Verification items for the finished model (mm, model axes). A direction names the side the tool comes from. Coordinates: 2 decimals unless noted, no trailing zeros. Write each loop counter-clockwise with the first axis right and the second up, starting at its lowest first coordinate (ties: lowest second). Pieces come first, ordered by that corner, then holes. Notation, with made-up numbers: M 5.25,-33 L 43.25,-33 A31 cw 43.25,-7 Z; hole C -26,-12.5 d4. An arc over 180 degrees is marked long. Answer in a Markdown table with one row per item.
from build123d import *

# Parameters (mm, degrees)
PAD_DEPTH       = 40
POCKET_DEPTH    = 35
POCKET001_DEPTH = 5
FILLET_R        = 0.5
FILLET001_R     = 0.5
CHAMFER_SIZE    = 1


with BuildPart() as part:
    # Sketch → Pad (new body)
    with BuildSketch(Plane.XY):
        with BuildLine():
            Line((-25, 20), (25, 20))
            ThreePointArc((30, 15), (28.535534, 18.535534), (25, 20))
            Line((30, 15), (30, -15))
            ThreePointArc((25, -20), (28.535534, -18.535534), (30, -15))
            Line((25, -20), (-25, -20))
            ThreePointArc((-30, -15), (-28.535534, -18.535534), (-25, -20))
            Line((-30, -15), (-30, 15))
            ThreePointArc((-25, 20), (-28.535534, 18.535534), (-30, 15))
        make_face()
    extrude(amount=PAD_DEPTH)

    # Sketch001 (on Face10 of Pad) → Pocket (cut)
    with BuildSketch(Plane.XY.offset(40)):
        with BuildLine():
            Line((-22.5, 17.5), (22.5, 17.5))
            ThreePointArc((27.5, 12.5), (26.035534, 16.035534), (22.5, 17.5))
            Line((27.5, 12.5), (27.5, -12.5))
            ThreePointArc((22.5, -17.5), (26.035534, -16.035534), (27.5, -12.5))
            Line((22.5, -17.5), (-22.5, -17.5))
            ThreePointArc((-27.5, -12.5), (-26.035534, -16.035534), (-22.5, -17.5))
            Line((-27.5, -12.5), (-27.5, 12.5))
            ThreePointArc((-22.5, 17.5), (-26.035534, 16.035534), (-27.5, 12.5))
        make_face()
    extrude(amount=-POCKET_DEPTH, mode=Mode.SUBTRACT)

    # Sketch002 (on Face6 of Pocket) → Pocket001 (cut)
    with BuildSketch(Plane.XZ.offset(20)):
        with BuildLine():
            Line((-13.5, 40), (13.5, 40))
            Line((13.5, 40), (13.5, 28.982013))
            ThreePointArc((11, 26.482013), (12.767767, 27.214246), (13.5, 28.982013))
            Line((11, 26.482013), (-11, 26.482013))
            ThreePointArc((-13.5, 28.982013), (-12.767767, 27.214246), (-11, 26.482013))
            Line((-13.5, 28.982013), (-13.5, 40))
        make_face()
    extrude(amount=-POCKET001_DEPTH, mode=Mode.SUBTRACT)

    # Fillet
    fillet_edges = [part.edges().sort_by_distance(p)[0] for p in [
        (13.5, -17.5, 34.491006),
        (12.767767, -17.5, 27.214246),
        (0, -17.5, 26.482013),
        (-12.767767, -17.5, 27.214246),
        (-13.5, -17.5, 34.491006),
        (-18, -17.5, 40),
        (-26.035534, -16.035534, 40),
        (-27.5, 0, 40),
        (-26.035534, 16.035534, 40),
        (0, 17.5, 40),
        (26.035534, 16.035534, 40),
        (27.5, 0, 40),
        (26.035534, -16.035534, 40),
        (18, -17.5, 40),
    ]]
    fillet(fillet_edges, radius=FILLET_R)

    # Fillet001
    fillet001_edges = [part.edges().sort_by_distance(p)[0] for p in [
        (-19.25, -20, 40),
        (-13.5, -20, 34.491006),
        (-12.767767, -20, 27.214246),
        (0, -20, 26.482013),
        (12.767767, -20, 27.214246),
        (13.5, -20, 34.491006),
        (19.25, -20, 40),
        (28.535534, -18.535534, 40),
        (30, 0, 40),
        (28.535534, 18.535534, 40),
        (0, 20, 40),
        (-28.535534, 18.535534, 40),
        (-30, 0, 40),
        (-28.535534, -18.535534, 40),
    ]]
    fillet(fillet001_edges, radius=FILLET001_R)

    # Chamfer
    chamfer_edges = [part.edges().sort_by_distance(p)[0] for p in [
        (0, -20, 0),
        (28.535534, -18.535534, 0),
        (30, 0, 0),
        (28.535534, 18.535534, 0),
        (0, 20, 0),
        (-28.535534, 18.535534, 0),
        (-30, 0, 0),
        (-28.535534, -18.535534, 0),
    ]]
    chamfer(chamfer_edges, length=CHAMFER_SIZE)


solid = part.part
1) Release check for a two-part mould opening along Y. For faces 4 (the face through (0, 0, 0)), 5 (the face through (-26.07, -16, 22.49)), 6 (the face through (-29, -18, 20)) record: +Y half, -Y half, draft (parallel to the pull), parting line (faces both ways), or undercut.
Response values:
| item | result |
|---|---|
| face 4 | draft |
| face 5 | undercut |
| face 6 | -Y half |
2) Sectioned sample at A-A (z = 20). Record the cut outline in (x, y), then the cut area to 3 significant figures.
Response values:
| item | result |
|---|---|
| outline | M -30,-15 A5 ccw -25,-20 L 25,-20 A5 ccw 30,-15 L 30,15 A5 ccw 25,20 L -25,20 A5 ccw -30,15 Z; hole M -27.5,-12.5 A5 ccw -22.5,-17.5 L 22.5,-17.5 A5 ccw 27.5,-12.5 L 27.5,12.5 A5 ccw 22.5,17.5 L -22.5,17.5 A5 ccw -27.5,12.5 Z |
| area | 475 mm² |
3) Sectioned sample at C-C (x = -17.5). Record the cut outline in (y, z), then the cut area to 3 significant figures.
Response values:
| item | result |
|---|---|
| outline | M -20,1 L -19,0 L 19,0 L 20,1 L 20,39.5 A0.5 ccw 19.5,40 L 18,40 A0.5 ccw 17.5,39.5 L 17.5,5 L -17.5,5 L -17.5,39.5 A0.5 ccw -18,40 L -19.5,40 A0.5 ccw -20,39.5 Z |
| area | 374 mm² |
4) Sectioned sample at D-D (z = 32). Record the cut outline in (x, y).
Response values:
| item | result |
|---|---|
| outline | M -30,-15 A5 ccw -25,-20 L -14,-20 A0.5 ccw -13.5,-19.5 L -13.5,-18 A0.5 ccw -14,-17.5 L -22.5,-17.5 A5 cw -27.5,-12.5 L -27.5,12.5 A5 cw -22.5,17.5 L 22.5,17.5 A5 cw 27.5,12.5 L 27.5,-12.5 A5 cw 22.5,-17.5 L 14,-17.5 A0.5 ccw 13.5,-18 L 13.5,-19.5 A0.5 ccw 14,-20 L 25,-20 A5 ccw 30,-15 L 30,15 A5 ccw 25,20 L -25,20 A5 ccw -30,15 Z |
5) Sectioned sample at B-B (y = -0.5). Record the cut outline in (x, z).
Response values:
| item | result |
|---|---|
| outline | M -30,1 L -29,0 L 29,0 L 30,1 L 30,39.5 A0.5 ccw 29.5,40 L 28,40 A0.5 ccw 27.5,39.5 L 27.5,5 L -27.5,5 L -27.5,39.5 A0.5 ccw -28,40 L -29.5,40 A0.5 ccw -30,39.5 Z |
6) Thickness scan on L1, parallel to X at y = -1, z = 33.5; L2, parallel to Y at x = 9, z = 17.5; L3, parallel to Z at x = 5.5, y = -9. Record the ranges inside material, lowest first. Write a range as [from, to].
Response values:
| item | result |
|---|---|
| L1 | x = [-30, -27.5], [27.5, 30] |
| L2 | y = [-20, -17.5], [17.5, 20] |
| L3 | z = [0, 5] |
7) Depth check by flat-ended pin: pin 1 (10 mm diameter, centred on x = -7.5, y = 6, fed in from +Z); pin 2 (1.6 mm diameter, centred on y = -19, z = 34.5, fed in from +X); pin 3 (0.8 mm diameter, centred on y = -18.5, z = 36.5, fed in from -X). Enter the tip coordinate at first touch or a pass-through.
Response values:
| item | result |
|---|---|
| pin 1 | stops at z = 5 |
| pin 2 | stops at x = 28.84 |
| pin 3 | stops at x = -28.92 |
8) Tool access check on faces 1 (the face through (-27.5, 0, 22)), 2 (the face through (-12.787, -18.76, 27.234)), 3 (the face through (-28, 19, 20)). Record the directions out of +Z, -Z, +X, -X, +Y, -Y that give a thin tool (end or side, any length) a straight path to the whole face; none if there is none.
Response values:
| item | result |
|---|---|
| face 1 | +Z |
| face 2 | +Z, -Y |
| face 3 | +Z, -Z, -X, +Y |
